Part model, mm, in its own coordinate system. Coordinates: 2 decimals unless noted, no trailing zeros. Write each loop counter-clockwise with the first axis right and the second up, starting at its lowest first coordinate (ties: lowest second). Pieces come first, ordered by that corner, then holes. Notation, with made-up numbers: (-23.5, 4.5) - (14.5, 4.5) arc R21 ccw to (14.5, 21.5) - close; hole circle Ø11 at (48.5, -18.75). An arc over 180 degrees is marked (long way). Use one line per item in the form item = value. Start each with the question number.
from build123d import *

# Parameters (mm, degrees)
SKETCH1_R          = 34.925
EXTRUDE1_DEPTH     = 19.05
SKETCH2_R          = 12.7
CUT_EXTRUDE1_DEPTH = 53.937829102
SKETCH3_R          = 3.3655
CUT_EXTRUDE2_DEPTH = 53.937829102
CIRPATTERN1_COUNT  = 6


with BuildPart() as part:
    # Sketch1 → Extrude1 (new body)
    with BuildSketch(Plane(origin=(0, 0, 0), x_dir=(1, 0, 0), z_dir=(0, 1, 0))):
        with Locations(Location((0, 0, 0), (0, 0, 90))):
            Circle(SKETCH1_R)
    extrude(amount=EXTRUDE1_DEPTH)

    # Sketch2 → Cut-Extrude1 (cut, through all)
    with BuildSketch(Plane(origin=(0, 0, 0), x_dir=(1, 0, 0), z_dir=(0, 1, 0))):
        with Locations(Location((0, 0, 0), (0, 0, 90))):
            Circle(SKETCH2_R)
    extrude(amount=CUT_EXTRUDE1_DEPTH, mode=Mode.SUBTRACT)

    # Sketch3 → Cut-Extrude2 (cut, through all)
    with BuildSketch(Plane(origin=(0, 0, 0), x_dir=(1, 0, 0), z_dir=(0, 1, 0))):
        with Locations(Location((0, 29.337, 0), (0, 0, 90))):
            Circle(SKETCH3_R)
    cut_extrude2 = extrude(amount=CUT_EXTRUDE2_DEPTH, mode=Mode.SUBTRACT)

    # CirPattern1: Cut-Extrude2 ×6 about axis
    cirpattern1_axis = Axis((0, 0, 0), (0, 1, 0))
    for i in range(1, CIRPATTERN1_COUNT):
        add(cut_extrude2.rotate(cirpattern1_axis, i * 360 / CIRPATTERN1_COUNT), mode=Mode.SUBTRACT)


solid = part.part
Q1. Slice it at A-A (z = 0). List the corners of the cut face in (x, y) (3 decimals), plus the area to 3 significant figures.
Q2. Slice it at C-C (x = 27.5). List the corners of the cut face in (y, z), plus the area to 3 significant figures.
Q3. Slice it at B-B (x = 0). Count the separate pieces of the cut face and the enclosed holes in it, plus the area to 3 significant figures.
Q4. Mould opens along X. For faces 1 (the flat face through (0, 0, -15)), 2 (the cylindrical face through (34.094, 9.392, 7.571)), 3 (the cylindrical face through (-2.275, 9.392, -26.856)) say: released by +X, released by -X, zero draft, split by the parting line, or undercut.
Q5. Pin check, flat tips, straight feed: P1, Ø10, axis at x = -27, y = 8, coming from the +Z side; P2, Ø5, axis at y = 5, z = 6.5, coming from the +X side; P3, Ø6, axis at y = 12.5, z = -11.5, coming from the +X side. Stop position of each tip, or through.
Q6. Drill centre lines: probe 1 along Z at (x, y) = (25.5, 12.5); probe 2 along X at (y, z) = (13, -13); probe 3 along Z at (x, y) = (-23, 5.5). Where is each one in solid material? Low to high.
Solution:
q1.outline = (-34.925, 0) - (-12.7, 0) - (-12.7, 19.05) - (-34.925, 19.05) - close; (12.7, 0) - (34.925, 0) - (34.925, 19.05) - (12.7, 19.05) - close
q1.area = 847 mm2
q2.outline = (0, -21.53) - (19.05, -21.53) - (19.05, -17.3) - (0, -17.3) - close; (0, -12.03) - (19.05, -12.03) - (19.05, 12.03) - (0, 12.03) - close; (0, 17.3) - (19.05, 17.3) - (19.05, 21.53) - (0, 21.53) - close
q2.area = 619 mm2
q3.separate_pieces = 4
q3.enclosed_holes = 0
q3.area = 590 mm2
q4.face_1 = zero draft
q4.face_2 = split by the parting line
q4.face_3 = undercut
q5.P1 = 27.12
q5.P2 = 34.7
q5.P3 = 33.87
q6.probe_1 = -23.86 to -18.03, -11.3 to 11.3, 18.03 to 23.86
q6.probe_2 = -32.42 to -28.33, -22.48 to 22.48, 28.33 to 32.42
q6.probe_3 = -26.28 to -17.02, -12.32 to 12.32, 17.02 to 26.28
